```python
from build123d import *

# Parameters (mm, degrees)
PAD_DEPTH       = 17
SKETCH001_W     = 17
SKETCH001_H     = 13
POCKET_DEPTH    = 17
POCKET001_DEPTH = 3
POCKET002_DEPTH = 3
PAD001_DEPTH    = 1
PAD002_DEPTH    = 1


with BuildPart() as part:
    # Sketch → Pad (new body)
    with BuildSketch(Plane.YZ):
        Polygon((0, 0), (0, 20), (-3, 20), (-20, 3), (-20, 0), align=None)
    extrude(amount=PAD_DEPTH)

    # Sketch001 (on Face4 of Pad) → Pocket (cut)
    with BuildSketch(Plane(origin=(0, -20, 0), x_dir=(0, 0, -1), z_dir=(0, -1, 0))):
        with Locations((-11.5, 8.5)):
            Rectangle(SKETCH001_W, SKETCH001_H)
    extrude(amount=-POCKET_DEPTH, mode=Mode.SUBTRACT)

    # Sketch002 (on Face8 of Pocket) → Pocket001 (cut)
    with BuildSketch(Plane(origin=(0, -3, 0), x_dir=(0, 0, -1), z_dir=(0, -1, 0))):
        with BuildLine():
            ThreePointArc((-10, 5.5), (-7, 8.5), (-10, 11.5))
            Line((-10, 11.5), (-13, 11.5))
            ThreePointArc((-13, 11.5), (-16, 8.5), (-13, 5.5))
            Line((-10, 5.5), (-13, 5.5))
        make_face()
    extrude(amount=-POCKET001_DEPTH, mode=Mode.SUBTRACT)

    # Sketch003 (on Face14 of Pocket001) → Pocket002 (cut)
    with BuildSketch(Plane(origin=(0, 0, 3), x_dir=(0, -1, 0), z_dir=(0, 0, 1))):
        with BuildLine():
            ThreePointArc((10, 11.5), (7, 8.5), (10, 5.5))
            Line((10, 5.5), (13, 5.5))
            ThreePointArc((13, 5.5), (16, 8.5), (13, 11.5))
            Line((10, 11.5), (13, 11.5))
        make_face()
    extrude(amount=-POCKET002_DEPTH, mode=Mode.SUBTRACT)

    # Sketch004 (on Face1 of Pocket002) → Pad001 (join)
    with BuildSketch(Plane.ZX):
        with BuildLine():
            ThreePointArc((4, 9.5), (3, 10.5), (2, 9.5))
            Line((2, 9.5), (2, 7.5))
            ThreePointArc((2, 7.5), (3, 6.5), (4, 7.5))
            Line((4, 9.5), (4, 7.5))
        make_face()
        with BuildLine():
            ThreePointArc((19, 9.5), (18, 10.5), (17, 9.5))
            Line((17, 9.5), (17, 7.5))
            ThreePointArc((17, 7.5), (18, 6.5), (19, 7.5))
            Line((19, 9.5), (19, 7.5))
        make_face()
    extrude(amount=PAD001_DEPTH)

    # Sketch005 (on Face2 of Pad001) → Pad002 (join)
    with BuildSketch(Plane.YX):
        with BuildLine():
            ThreePointArc((-4, 7.5), (-3, 6.5), (-2, 7.5))
            Line((-2, 7.5), (-2, 9.5))
            ThreePointArc((-2, 9.5), (-3, 10.5), (-4, 9.5))
            Line((-4, 7.5), (-4, 9.5))
        make_face()
        with BuildLine():
            ThreePointArc((-17, 9.5), (-18, 10.5), (-19, 9.5))
            Line((-19, 9.5), (-19, 7.5))
            ThreePointArc((-19, 7.5), (-18, 6.5), (-17, 7.5))
            Line((-17, 9.5), (-17, 7.5))
        make_face()
    extrude(amount=PAD002_DEPTH)


solid = part.part
```
Build history of the part. All positions in model axes, mm. A direction names the side the tool comes from. Round coordinates to 2 decimals unless told otherwise and drop trailing zeros. Order: outer loops, then holes, each group sorted by start corner. A loop starts at its lowest first (then second) coordinate and runs counter-clockwise, first axis right, second up. Notation, with made-up numbers: (14, -19.75) - (34, -19.75) arc R15 ccw to (34, -11.75) - close; hole circle Ø11 at (7, 50.5). An arc over 180 degrees is marked (long way). Use a Markdown table: item, result.
1) Saw through at B-B on y = -1.25. Write the cut outline in (x, z).
Recorded:
| item | result |
|---|---|
| outline | (0, 0) - (17, 0) - (17, 20) - (0, 20) - close; hole (5.5, 10) arc R3 ccw to (11.5, 10) - (11.5, 13) arc R3 ccw to (5.5, 13) - close |
2) Saw through at A-A on y = -11.25. Write the cut outline in (x, z).
Recorded:
| item | result |
|---|---|
| outline | (0, 0) - (5.5, 0) - (5.5, 3) - (2, 3) - (2, 11.75) - (0, 11.75) - close; (11.5, 0) - (17, 0) - (17, 11.75) - (15, 11.75) - (15, 3) - (11.5, 3) - close |
3) Saw through at C-C on z = 13.5. Write the cut outline in (x, y).
Recorded:
| item | result |
|---|---|
| outline | (0, -9.5) - (2, -9.5) - (2, -3) - (5.54, -3) - (5.54, 0) - (0, 0) - close; (11.46, -3) - (15, -3) - (15, -9.5) - (17, -9.5) - (17, 0) - (11.46, 0) - close |
4) Saw through at D-D on x = 8. Give the number of separate pieces and of enclosed holes in the cut face, and give its area (3 significant figures).
Recorded:
| item | result |
|---|---|
| separate pieces | 3 |
| enclosed holes | 0 |
| area | 65.5 mm² |
5) Flat gauge pins, fed straight in: pin 1 Ø3 at (x, z) = (5, 8.5) entering from +Y; pin 2 Ø0.8 at (x, y) = (8.5, 0.5) entering from -Z; pin 3 Ø1.5 at (x, y) = (5, -6) entering from +Z; pin 4 Ø2 at (y, z) = (-18, 7.5) entering from +X. Where does each tip first touch, or does it go through?
Recorded:
| item | result |
|---|---|
| pin 1 | stops at y = 0 |
| pin 2 | stops at z = 2 |
| pin 3 | stops at z = 3 |
| pin 4 | passes through |
6) Tool access for faces 5 (the face through (5.5, -11, 2)), 6 (the face through (6.5, 0.5, 3)), 7 (the face through (8.5, -2, -0.5)), 8 (the face through (8.6, -1.5, 16)), 9 (the face through (8.5, -19, -0.5)): list every direction of +Z, -Z, +X, -X, +Y, -Y with a clear straight run to the whole face (end or side of a thin tool).
Recorded:
| item | result |
|---|---|
| face 5 | +Z, -Z |
| face 6 | -X, +Y |
| face 7 | -Z, +X, -X, +Y |
| face 8 | +Y, -Y |
| face 9 | -Z, +X, -X, -Y |
7) Wall check: L1, parallel to X at y = -10.25, z = 4.25; L2, parallel to Y at x = 3.5, z = 6.5; L3, parallel to Z at x = 14.75, y = -7.25. Give the ranges that are in metal, low to high.
Recorded:
| item | result |
|---|---|
| L1 | x = 0 to 2, 15 to 17 |
| L2 | y = -3 to 0 |
| L3 | z = 0 to 3 |
8) Pull direction Z, two halves, no side cores. Call faces 1 (the face through (1, -11, 12)), 2 (the face through (8.6, -7, 1.5)), 3 (the face through (6.5, 0.5, 18)), 4 (the face through (10.5, 0.5, 3)): pulls with the +Z half, pulls with the -Z half, needs draft (parallel to the pull), parting line crosses it, or undercut.
Recorded:
| item | result |
|---|---|
| face 1 | pulls with the +Z half |
| face 2 | needs draft |
| face 3 | undercut |
| face 4 | undercut |
